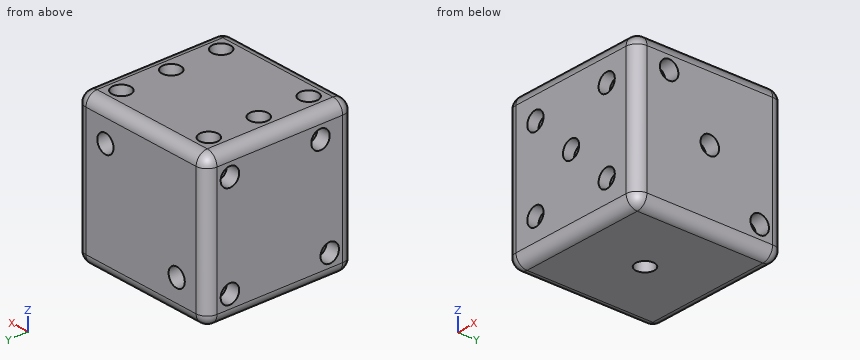
from build123d import *

# Parameters (mm, degrees)
F0_W      = 20
F0_H      = 20
F1_DEPTH  = 20
F2_R      = 1.5
F3_R      = 1.25
F4_DEPTH  = 2
F5_R      = 1.25
F6_DEPTH  = 1.5
F7_R      = 1.25
F8_DEPTH  = 2
F9_R      = 1.25
F10_DEPTH = 1.9
F11_R     = 1.25
F12_DEPTH = 1.9
F13_R     = 1.25
F14_DEPTH = 2


with BuildPart() as f1:
    # F0 (on Top) → F1 (new body)
    with BuildSketch(Plane.XY):
        Rectangle(F0_W, F0_H)
    extrude(amount=F1_DEPTH)

    # F2
    f2_edges = [f1.edges().sort_by_distance(p)[0] for p in [
        (10, 10, 10),
        (-10, 10, 10),
        (0, 10, 0),
        (0, 10, 20),
        (-10, -10, 10),
        (10, -10, 10),
        (0, -10, 0),
        (0, -10, 20),
        (-10, 0, 20),
        (10, 0, 20),
        (10, 0, 0),
        (-10, 0, 0),
    ]]
    fillet(f2_edges, radius=F2_R)

    # F3 (on face) → F4 (cut)
    with BuildSketch(Plane.YZ.offset(10)):
        with Locations((-5.5, 16.75)):
            Circle(F3_R)
        with Locations((0, 10)):
            Circle(F3_R)
        with Locations((6.75, 3.25)):
            Circle(F3_R)
    extrude(amount=-F4_DEPTH, mode=Mode.SUBTRACT)

    # F5 (on face) → F6 (cut)
    with BuildSketch(Plane.XZ.offset(10)):
        with Locations((-5.5, 4.5)):
            Circle(F5_R)
        with Locations((5.5, 15.5)):
            Circle(F5_R)
        with Locations((-5.5, 15.5)):
            Circle(F5_R)
        with Locations((0, 10)):
            Circle(F5_R)
        with Locations((5.5, 4.5)):
            Circle(F5_R)
    extrude(amount=-F6_DEPTH, mode=Mode.SUBTRACT)

    # F7 (on face) → F8 (cut)
    with BuildSketch(Plane(origin=(0, 10, 0), x_dir=(-1, 0, 0), z_dir=(0, 1, 0))):
        with Locations((-5.5, 15.5)):
            Circle(F7_R)
        with Locations((5.5, 4.5)):
            Circle(F7_R)
    extrude(amount=-F8_DEPTH, mode=Mode.SUBTRACT)

    # F9 (on face) → F10 (cut)
    with BuildSketch(Plane(origin=(-10, 0, 0), x_dir=(0, -1, 0), z_dir=(-1, 0, 0))):
        with Locations((-6.75, 3.25)):
            Circle(F9_R)
        with Locations((5.5, 16.75)):
            Circle(F9_R)
        with Locations((6.75, 3.25)):
            Circle(F9_R)
        with Locations((-6.75, 16.75)):
            Circle(F9_R)
    extrude(amount=-F10_DEPTH, mode=Mode.SUBTRACT)

    # F11 (on face) → F12 (cut)
    with BuildSketch(Plane.XY.offset(20)):
        with Locations((-6.75, 6.75)):
            Circle(F11_R)
        with Locations((-6.75, -6.75)):
            Circle(F11_R)
        with Locations((-6.75, 0)):
            Circle(F11_R)
        with Locations((6.75, 6.75)):
            Circle(F11_R)
        with Locations((6.75, 0)):
            Circle(F11_R)
        with Locations((6.75, -6.75)):
            Circle(F11_R)
    extrude(amount=-F12_DEPTH, mode=Mode.SUBTRACT)

    # F13 (on face) → F14 (cut)
    with BuildSketch(Plane(origin=(0, 0, 0), x_dir=(1, 0, 0), z_dir=(0, 0, -1))):
        Circle(F13_R)
    extrude(amount=-F14_DEPTH, mode=Mode.SUBTRACT)


solid = f1.part
Design review of the part built by this model. Coordinates are the model's own, in mm. Give positions to 0.01 mm unless a question says otherwise; leave off trailing zeros. Order: outer loops, then holes, each group sorted by start corner. A loop starts at its lowest first (then second) coordinate and runs counter-clockwise, first axis right, second up.
1. Add section C-C, the plane x = 0. State the section outline as (y, z) points, then the cut area to 3 significant figures.
Solution:
outline: (-10, 1.5) arc R1.5 ccw to (-8.5, 0) - (-1.25, 0) - (-1.25, 2) - (1.25, 2) - (1.25, 0) - (8.5, 0) arc R1.5 ccw to (10, 1.5) - (10, 18.5) arc R1.5 ccw to (8.5, 20) - (-8.5, 20) arc R1.5 ccw to (-10, 18.5) - (-10, 11.25) - (-8.5, 11.25) - (-8.5, 8.75) - (-10, 8.75) - close
area: 389 mm2
2. Add section A-A, the plane y = 6.75. State the section outline as (x, z) points, then the cut area to 3 significant figures.
Solution:
outline: (-10, 1.5) arc R1.5 ccw to (-8.5, 0) - (8.5, 0) arc R1.5 ccw to (10, 1.5) - (10, 2) - (8, 2) - (8, 4.5) - (10, 4.5) - (10, 18.5) arc R1.5 ccw to (8.5, 20) - (8, 20) - (8, 18.1) - (5.5, 18.1) - (5.5, 20) - (-5.5, 20) - (-5.5, 18.1) - (-8, 18.1) - (-8, 20) - (-8.5, 20) arc R1.5 ccw to (-10, 18.5) - (-10, 18) - (-8.1, 18) - (-8.1, 15.5) - (-10, 15.5) - (-10, 4.5) - (-8.1, 4.5) - (-8.1, 2) - (-10, 2) - close
area: 374 mm2
3. To check wall thickness, follow L1, parallel to X at y = -9, z = 4; L2, parallel to Z at x = 5.75, y = -9; L3, parallel to Y at x = -6.75, z = 19.15. State the ranges of each line that lie inside material, in increasing order.
Solution:
L1: x = -9.91 to -6.65, -4.35 to 4.35, 6.65 to 9.91
L2: z = 0.09 to 3.28, 5.72 to 14.28, 16.72 to 19.91
L3: y = -9.85 to -8, -5.5 to -1.25, 1.25 to 5.5, 8 to 9.85
4. For pin 1 Ø0.8 at (x, z) = (5, 4.5) entering from -Y; pin 2 Ø1.5 at (y, z) = (-5.5, 16.75) entering from +X; pin 3 Ø1.5 at (x, y) = (6.75, 0) entering from +Z, all flat-tipped, find the tip position at first contact; note any pin that passes through.
Solution:
pin 1: stops at y = -8.5
pin 2: stops at x = 8
pin 3: stops at z = 18.1
5. Add section B-B, the plane z = 10. State the section outline as (x, y) points, then the cut area to 3 significant figures.
Solution:
outline: (-10, -8.5) arc R1.5 ccw to (-8.5, -10) - (-1.25, -10) - (-1.25, -8.5) - (1.25, -8.5) - (1.25, -10) - (8.5, -10) arc R1.5 ccw to (10, -8.5) - (10, -1.25) - (8, -1.25) - (8, 1.25) - (10, 1.25) - (10, 8.5) arc R1.5 ccw to (8.5, 10) - (-8.5, 10) arc R1.5 ccw to (-10, 8.5) - close
area: 389 mm2
